```python
from build123d import *

# Parameters (mm, degrees)
SM_BASE_FLANGE_1_DEPTH           = 1.5
SM_EDGE_FLANGE_1_STRIP_W         = 7.4732
SM_EDGE_FLANGE_1_STRIP_H         = 1.5
SM_EDGE_FLANGE_1_STRIP_CUT_DEPTH = 40
SM_EDGE_FLANGE_1_DEPTH           = 40
CUT_EXTRUDE_1_DEPTH              = 10
SKETCH_10_R                      = 1.6
CUT_EXTRUDE_2_DEPTH              = 10
SKETCH_11_R                      = 1.75
CUT_EXTRUDE_3_DEPTH              = 10


# Sheet-metal steps are written as plain solids
with BuildPart() as part:
    # Sketch 1 → 基体-法兰1 (new body)
    with BuildSketch(Plane(origin=(0, 0, 0), x_dir=(1, 0, 0), z_dir=(0, 1, 0))):
        with BuildLine():
            Line((-17, -20), (17, -20))
            ThreePointArc((17, -20), (19.121320344, -19.121320344), (20, -17))
            Line((20, -17), (20, 20))
            Line((20, 20), (-20, 20))
            Line((-20, 20), (-20, -17))
            ThreePointArc((-20, -17), (-19.121320344, -19.121320344), (-17, -20))
        make_face()
    extrude(amount=-SM_BASE_FLANGE_1_DEPTH)

    # 边线-法兰1 strip (across the edge) → 边线-法兰1 strip cut (cut)
    with BuildSketch(Plane(origin=(20, 0, -20), x_dir=(0, 0, 1), z_dir=(-1, 0, 0))):
        with Locations((-3, -0.75)):
            Rectangle(SM_EDGE_FLANGE_1_STRIP_W, SM_EDGE_FLANGE_1_STRIP_H)
    extrude(amount=SM_EDGE_FLANGE_1_STRIP_CUT_DEPTH, mode=Mode.SUBTRACT)

    # 边线-法兰1 section (across the edge) → 边线-法兰1 (add)
    with BuildSketch(Plane(origin=(20, 0, -20), x_dir=(0, 0, 1), z_dir=(-1, 0, 0))):
        with BuildLine():
            Line((-1.5, 0.7366), (-1.5, 44.5))
            Line((-1.5, 44.5), (0, 44.5))
            Line((0, 44.5), (0, 0.7366))
            ThreePointArc((0, 0.7366), (0.215745145, 0.215745145), (0.7366, 0))
            Line((0.7366, 0), (0.7366, -1.5))
            ThreePointArc((0.7366, -1.5), (-0.844915027, -0.844915027), (-1.5, 0.7366))
        make_face()
    extrude(amount=SM_EDGE_FLANGE_1_DEPTH)

    # 草图9 → 切除-拉伸1 (cut)
    with BuildSketch(Plane(origin=(0, 0, -21.5), x_dir=(-1, 0, 0), z_dir=(0, 0, -1))):
        with BuildLine():
            Line((-20, 24.5), (-20, 44.5))
            Line((-20, 44.5), (25.146997012, 48.516846867))
            Line((25.146997012, 48.516846867), (20, 24.5))
            ThreePointArc((20, 24.5), (0, 44.5), (-20, 24.5))
        make_face()
    extrude(amount=-CUT_EXTRUDE_1_DEPTH, mode=Mode.SUBTRACT)

    # 草图10 → 切除-拉伸2 (cut)
    with BuildSketch(Plane(origin=(0, 0, -21.5), x_dir=(-1, 0, 0), z_dir=(0, 0, -1))):
        with Locations(Location((7.75, 37.923393759, 0), (0, 0, 90))):
            Circle(SKETCH_10_R)
        with Locations(Location((15.5, 24.5, 0), (0, 0, 90))):
            Circle(SKETCH_10_R)
        with Locations(Location((7.75, 11.076606241, 0), (0, 0, 90))):
            Circle(SKETCH_10_R)
        with Locations(Location((-7.75, 11.076606241, 0), (0, 0, 90))):
            Circle(SKETCH_10_R)
        with Locations(Location((-15.5, 24.5, 0), (0, 0, 90))):
            Circle(SKETCH_10_R)
        with Locations(Location((-7.75, 37.923393759, 0), (0, 0, 90))):
            Circle(SKETCH_10_R)
        with BuildLine():
            Line((-6.5, 17.5), (-6.5, 31.5))
            ThreePointArc((-6.5, 31.5), (0, 38), (6.5, 31.5))
            Line((6.5, 31.5), (6.5, 17.5))
            ThreePointArc((6.5, 17.5), (0, 11), (-6.5, 17.5))
        make_face()
    extrude(amount=-CUT_EXTRUDE_2_DEPTH, mode=Mode.SUBTRACT)

    # 草图11 → 切除-拉伸3 (cut)
    with BuildSketch(Plane.XZ.offset(1.5)):
        with Locations(Location((15, 12, 0), (0, 0, 270))):
            Circle(SKETCH_11_R)
        with Locations(Location((-15, 12, 0), (0, 0, 270))):
            Circle(SKETCH_11_R)
        with Locations(Location((-15, -12, 0), (0, 0, 270))):
            Circle(SKETCH_11_R)
        with Locations(Location((15, -12, 0), (0, 0, 270))):
            Circle(SKETCH_11_R)
    extrude(amount=-CUT_EXTRUDE_3_DEPTH, mode=Mode.SUBTRACT)


solid = part.part
```
Part model, mm, in its own coordinate system. A direction names the side the tool comes from. Coordinates: 2 decimals unless noted, no trailing zeros. Order: outer loops, then holes, each group sorted by start corner. A loop starts at its lowest first (then second) coordinate and runs counter-clockwise, first axis right, second up. Notation, with made-up numbers: (-29.75, 85) -> (0.25, 85) arc R27 ccw to (0.25, 101) -> close; hole circle Ø1 at (83, 2.5). An arc over 180 degrees is marked (long way). Put each result on its own line as item: value. Start each with the question number.
(1) Band-saw the part on B-B (x = -7.75). Give the cut face in (y, z).
(2) Pin check, flat tips, straight feed: pin 1 Ø3 at (x, z) = (-15, 12) entering from +Y; pin 2 Ø5 at (x, y) = (7.75, 11.08) entering from +Z; pin 3 Ø1.2 at (y, z) = (25.5, -21) entering from -X; pin 4 Ø5.5 at (x, z) = (15, 12) entering from +Y. Stop position of each tip, or through.
(3) Band-saw the part on C-C (x = 0). Give the cut face in (y, z).
(4) Which spindle directions (+Z, -Z, +X, -X, +Y, -Y) get a long thin tool onto all of the face, cutting with end or side? Do faces 1 (the face through (0, 0, 0)), 2 (the face through (-20, -1, -11)), 3 (the face through (0, 11, -21)). Say none if no direction does.
(5) Band-saw the part on D-D (y = 12). Give the cut face in (x, z).
(6) Probe line 1 along X through (y, z) = (-0.7, -12); line 2 along X through (y, z) = (24.5, -20.45); line 3 along Z through (x, y) = (10, 24.5). List the from-to ranges inside material, lowest first. Write a range as [from, to].
(7) Mould opens along Y. For faces 4 (the face through (0, 38, -21)), 5 (the face through (-9, 18, -20)), 6 (the face through (-13.914, 24.292, -20.76)), 7 (the face through (-0.44, 44.495, -20.76)) say: pulls with the +Y half, pulls with the -Y half, needs draft (parallel to the pull), parting line crosses it, or undercut.
(8) Band-saw the part on A-A (y = 20). Give the cut face in (x, z), then the cut area to 3 significant figures.
Determined:
1. outline: (-1.5, -19.26) arc R2.24 ccw to (0.74, -21.5) -> (9.48, -21.5) -> (9.48, -20) -> (0.74, -20) arc R0.74 cw to (0, -19.26) -> (0, 20) -> (-1.5, 20) -> close; (12.68, -21.5) -> (36.32, -21.5) -> (36.32, -20) -> (12.68, -20) -> close; (39.52, -21.5) -> (42.94, -21.5) -> (42.94, -20) -> (39.52, -20) -> close
2. pin 1: passes through
2. pin 2: stops at z = -20
2. pin 3: stops at x = -20
2. pin 4: stops at y = 0
3. outline: (-1.5, -19.26) arc R2.24 ccw to (0.74, -21.5) -> (11, -21.5) -> (11, -20) -> (0.74, -20) arc R0.74 cw to (0, -19.26) -> (0, 20) -> (-1.5, 20) -> close; (38, -21.5) -> (44.5, -21.5) -> (44.5, -20) -> (38, -20) -> close
4. face 1: +Z, +X, -X, +Y
4. face 2: +Z, -Z, -X, +Y, -Y
4. face 3: +Z, -Z
5. outline: (-20, -21.5) -> (-9.06, -21.5) -> (-9.06, -20) -> (-20, -20) -> close; (-6.44, -21.5) -> (-3.46, -21.5) -> (-3.46, -20) -> (-6.44, -20) -> close; (3.46, -21.5) -> (6.44, -21.5) -> (6.44, -20) -> (3.46, -20) -> close; (9.06, -21.5) -> (20, -21.5) -> (20, -20) -> (9.06, -20) -> close
6. line 1: x = [-20, -16.75], [-13.25, 13.25], [16.75, 20]
6. line 2: x = [-20, -17.1], [-13.9, -6.5], [6.5, 13.9], [17.1, 20]
6. line 3: z = [-21.5, -20]
7. face 4: undercut
7. face 5: needs draft
7. face 6: undercut
7. face 7: pulls with the +Y half
8. outline: (-20, -21.5) -> (-6.5, -21.5) -> (-6.5, -20) -> (-20, -20) -> close; (6.5, -21.5) -> (20, -21.5) -> (20, -20) -> (6.5, -20) -> close
8. area: 40.5 mm²
